The figure shows three views and two pictorial views of one solid part (mm, origin at its lowest corner). Answer the questions. A direction names the side the tool comes from. Coordinates: 2 decimals unless noted, no trailing zeros. Order: outer loops, then holes, each group sorted by start corner. A loop starts at its lowest first (then second) coordinate and runs counter-clockwise, first axis right, second up. Notation, with made-up numbers: (76.5, 32) - (91.5, 32) arc R21 cw to (91.5, 38) - close; hole circle Ø3 at (-27.5, 64). An arc over 180 degrees is marked (long way). Use one line per item in the form item = value. Start each with the question number.
Item 1: Section C-C, the plane x = 68 is taken. Write down the section's boundary in (y, z), and give its area (3 significant figures).
Item 2: A tool of negligible diameter and unlimited length cuts with its end or side. For the marked faces 5, 6 and 7, from which of +Z, -Z, +X, -X, +Y, -Y can it reach the whole face along a straight path? Write none if from no direction.
Item 3: Section A-A, the plane x = 40 is taken. Write down the section's boundary in (y, z).
Item 4: Section D-D, the plane x = 29.5 is taken. Write down the section's boundary in (y, z).
Item 5: Section B-B, the plane y = 32.5 is taken. Write down the section's boundary in (x, z), and give its area (3 significant figures).
Item 6: Consider line 1 along Y through (x, z) = (41, 9); line 2 along Z through (x, y) = (20, 65); line 3 along Z through (x, y) = (34.5, 59). Determine where each line is inside the solid, lowest interval first. Write a range as [from, to].
Item 7: The mould has two halves that part along X. Classify the marked faces 1, 2, 3 and 4: released by +X, released by -X, zero draft, split by the parting line, or undercut.
Item 8: Each of these flat-tipped pins is pushed along its axis until it touches: pin 1 Ø3 at (x, z) = (56.5, 1.5) entering from +Y; pin 2 Ø6.5 at (y, z) = (44, 7.5) entering from +X; pin 3 Ø4 at (y, z) = (55.5, 5.5) entering from -X; pin 4 Ø1 at (y, z) = (60.5, 3) entering from -X. Where does it stop, or does it pass through?
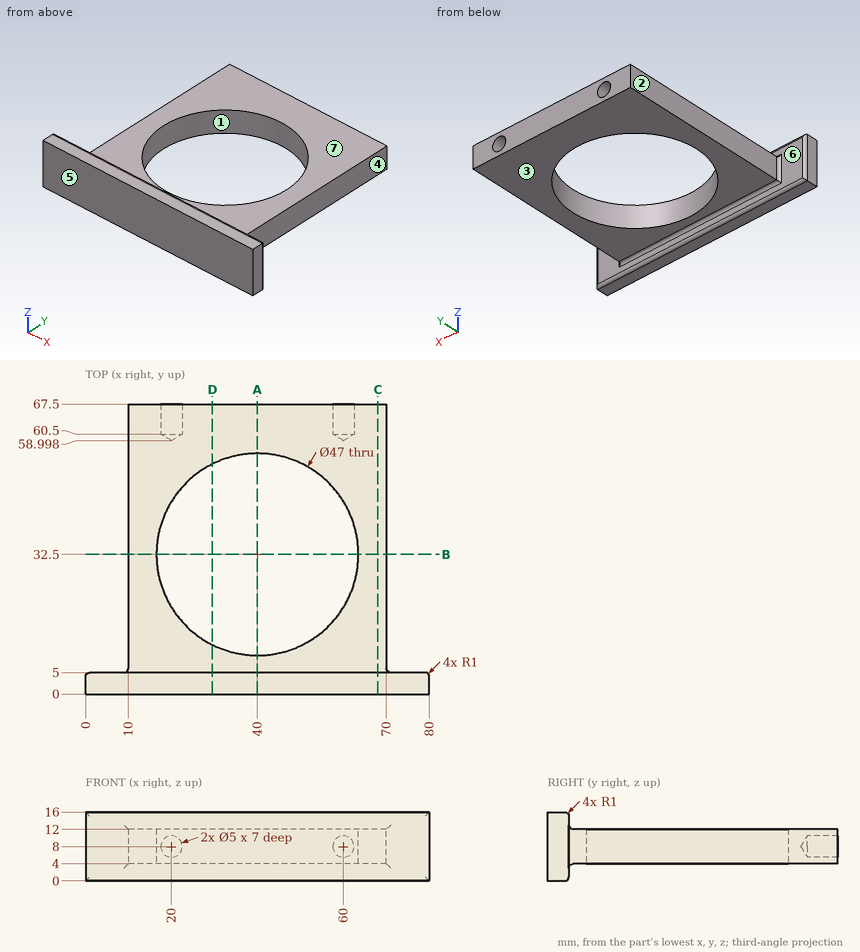
Response:
q1.outline = (0, 0) - (4, 0) arc R1 ccw to (5, 1) - (5, 3) arc R1 cw to (6, 4) - (67.5, 4) - (67.5, 12) - (6, 12) arc R1 cw to (5, 13) - (5, 15) arc R1 ccw to (4, 16) - (0, 16) - close
q1.area = 580 mm2
q2.face_5 = +Z, -Z, +X, -X, -Y
q2.face_6 = +Y
q2.face_7 = +Z, +X, -X, +Y
q3.outline = (0, 0) - (4, 0) arc R1 ccw to (5, 1) - (5, 3) arc R1 cw to (6, 4) - (9, 4) - (9, 12) - (6, 12) arc R1 cw to (5, 13) - (5, 15) arc R1 ccw to (4, 16) - (0, 16) - close; (56, 4) - (67.5, 4) - (67.5, 12) - (56, 12) - close
q4.outline = (0, 0) - (4, 0) arc R1 ccw to (5, 1) - (5, 3) arc R1 cw to (6, 4) - (11.48, 4) - (11.48, 12) - (6, 12) arc R1 cw to (5, 13) - (5, 15) arc R1 ccw to (4, 16) - (0, 16) - close; (53.52, 4) - (67.5, 4) - (67.5, 12) - (53.52, 12) - close
q5.outline = (10, 4) - (16.5, 4) - (16.5, 12) - (10, 12) - close; (63.5, 4) - (70, 4) - (70, 12) - (63.5, 12) - close
q5.area = 104 mm2
q6.line_1 = [0, 9.02], [55.98, 67.5]
q6.line_2 = [4, 5.5], [10.5, 12]
q6.line_3 = [4, 12]
q7.face_1 = undercut
q7.face_2 = released by -X
q7.face_3 = zero draft
q7.face_4 = released by +X
q8.pin_1 = 5
q8.pin_2 = 70
q8.pin_3 = 10
q8.pin_4 = through
